Design review of the part built by this model. Coordinates are the model's own, in mm. A direction names the side the tool comes from. Coordinates: 2 decimals unless noted, no trailing zeros. Loops run counter-clockwise (first coordinate to the right, second up) from the corner with the lowest first, then second, coordinate; pieces in that order, holes last. Notation, with made-up numbers: M -12,-31 L 2,-31 A33 cw 2,2 Z; hole C 58.5,64.25 d9. An arc over 180 degrees is marked long. Write item = value, one per line. Start each with the question number.
```python
from build123d import *

# Parameters (mm, degrees)
F1_DEPTH = 6.35


with BuildPart() as f1:
    # F0 (on Top) → F1 (new body)
    with BuildSketch(Plane.XY):
        Polygon((38.1, 3.96875), (38.1, 30.95625), (0, 30.95625), (-38.1, 30.95625), (-38.1, 3.96875), (-31.75, -19.84375), (0, -19.84375), (31.75, -19.84375), align=None)
        Polygon((-15.875, 10.31875), (0, 10.31875), (15.875, 10.31875), (15.875, -10.31875), (0, -10.31875), (-15.875, -10.31875), align=None, mode=Mode.SUBTRACT)
    extrude(amount=F1_DEPTH)


solid = f1.part
```
(1) To check wall thickness, follow L1, parallel to X at y = 9.5, z = 2.5 (3 decimals); L2, parallel to Y at x = 9.5, z = 3.5; L3, parallel to X at y = 3, z = 4.25 (3 decimals). State the ranges of each line that lie inside material, in increasing order.
(2) Take a section at D-D (y = -17). State the section outline as (x, z) points, plus the area to 3 significant figures.
(3) Insertion check: pin 1 (1.9 mm diameter, centred on y = 0.5, z = 3.5, fed in from -X); pin 2 (1.9 mm diameter, centred on y = -2, z = 4, fed in from +X). Each pin has a flat end and moves straight along its axis. Give the tip position at first contact, or say it passes through.
(4) Take a section at B-B (y = -6). State the section outline as (x, z) points (3 decimals).
(5) Take a section at C-C (y = 1.5). State the section outline as (x, z) points (3 decimals), plus the area to 3 significant figures.
(6) Take a section at A-A (z = 3.5). State the section outline as (x, y) points (3 decimals), plus the area to 3 significant figures.
(7) Mouldability with a two-part tool opening along X and no side actions: class faces 3 (the flat face through (0, -19.844, 3)), 4 (the flat face through (-38.1, 18, 3)), 5 (the flat face through (-15.875, 0, 3)), 6 (the flat face through (0, -10.319, 3)) as +X half, -X half, draft (parallel to the pull), parting line (faces both ways), or undercut.
(8) Tool access review of faces 1 (the flat face through (0, 10.319, 3)), 2 (the flat face through (-34.97, -7.77, 3.13)): name each direction out of +Z, -Z, +X, -X, +Y, -Y from which nothing blocks a thin tool from reaching the whole face with its end or side.
Results list:
q1.L1 = -38.1 to -15.875, 15.875 to 38.1
q1.L2 = -19.84 to -10.32, 10.32 to 30.96
q1.L3 = -37.842 to -15.875, 15.875 to 37.842
q2.outline = M -32.51,0 L 32.51,0 L 32.51,6.35 L -32.51,6.35 Z
q2.area = 413 mm^2
q3.pin_1 = -37.43
q3.pin_2 = 36.76
q4.outline = M -35.442,0 L -15.875,0 L -15.875,6.35 L -35.442,6.35 Z; M 15.875,0 L 35.442,0 L 35.442,6.35 L 15.875,6.35 Z
q5.outline = M -37.442,0 L -15.875,0 L -15.875,6.35 L -37.442,6.35 Z; M 15.875,0 L 37.442,0 L 37.442,6.35 L 15.875,6.35 Z
q5.area = 274 mm^2
q6.outline = M -38.1,3.969 L -31.75,-19.844 L 31.75,-19.844 L 38.1,3.969 L 38.1,30.956 L -38.1,30.956 Z; hole M -15.875,-10.319 L 15.875,-10.319 L 15.875,10.319 L -15.875,10.319 Z
q6.area = 3,060 mm^2
q7.face_3 = draft
q7.face_4 = -X half
q7.face_5 = undercut
q7.face_6 = undercut
q8.face_1 = +Z, -Z
q8.face_2 = +Z, -Z, -X, -Y
